Design review of the part built by this model. Coordinates are the model's own, in mm. Face numbers are marked on the shaded views. A direction names the side the tool comes from. Give positions to 0.01 mm unless a question says otherwise; leave off trailing zeros. Write each loop counter-clockwise with the first axis right and the second up, starting at its lowest first coordinate (ties: lowest second). Pieces come first, ordered by that corner, then holes.
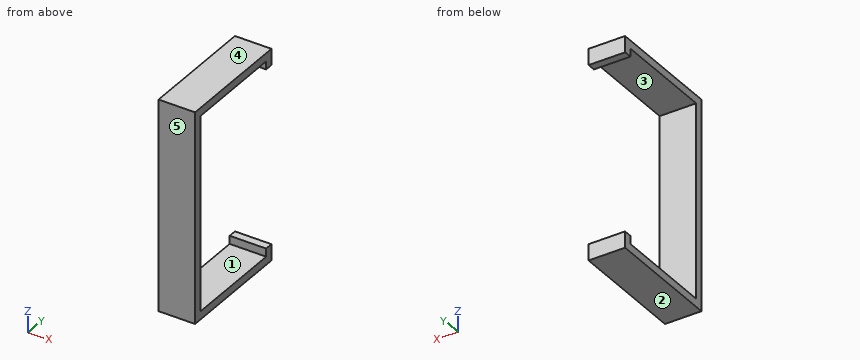
Autodesk Inventor part; units mm, degrees
ref_plane "YZ Plane" through (0, 0, 0) normal (1, 0, 0) x (0, 1, 0)
ref_plane "XZ Plane" through (0, 0, 0) normal (0, 1, 0) x (-1, 0, 0)
ref_plane "XY Plane" through (0, 0, 0) normal (0, 0, 1) x (1, 0, 0)
sketch "Skizze1" plane through (0, 0, 0) normal (0, 1, 0) x (-1, 0, 0)
  line L0 (0, 0) -> (12, 0)
  line L1 (12, 0) -> (12, -26)
  line L2 (12, -26) -> (0, -26)
  line L3 (0, -26) -> (0, 0)
  dimension "d0" = 12
  dimension "d1" = 26
extrude "Extrusion1" add sketch "Skizze1" along normal blind 1
sketch "Skizze2" plane through (0, 0, 0) normal (1, 0, 0) x (0, 0, -1)
  line L0 (26, 1) -> (0, 1)
  line L1 (0, 1) -> (0, 14.5)
  line L2 (0, 1) -> (13.5, 1) construction
  line L3 (0, 14.5) -> (2, 14.5)
  line L4 (2, 14.5) -> (2, 13.5)
  line L5 (2, 13.5) -> (1, 13.5)
  line L6 (1, 13.5) -> (1, 1)
  line L7 (0, 1) -> (1, 1)
  line L8 (24, 14.5) -> (26, 14.5)
  line L9 (26, 14.5) -> (26, 1)
  line L10 (26, 1) -> (25, 1)
  line L11 (25, 1) -> (25, 13.5)
  line L12 (25, 13.5) -> (24, 13.5)
  line L13 (24, 13.5) -> (24, 14.5)
  line L14 (25, 1) -> (26, 1)
  line L15 (26, 0) -> (26, 1)
  point P0 (0, 0)
  dimension "d4" = 13.5
  dimension "d5" = 90
  dimension "d6" = 2
  dimension "d7" = 1
  dimension "d8" = 1
  dimension "d9" = 2
  dimension "d10" = 24
  dimension "d11" = 1
  dimension "d12" = 13.5
  dimension "d13" = 0
extrude "Extrusion2" add sketch "Skizze2" against normal blind 12
sketch "Skizze3" plane through (-12, 0, 0) normal (0, 0, 1) x (1, 0, 0)
  line L0 (0, 0) -> (0, 14.5)
  line L1 (0, 0) -> (4, 0)
  line L2 (4, 0) -> (4, 1)
  line L3 (4, 1) -> (0, 1)
  line L4 (0, 1) -> (0, 0)
  line L5 (12, 14.5) -> (0, 14.5)
  line L6 (5, 14.5) -> (7.5, 14.5)
  line L7 (7.5, 14.5) -> (7.5, 1)
  line L8 (5, 14.5) -> (5, 1)
  line L9 (5, 1) -> (7.5, 1)
  line L10 (12, 0) -> (12, 14.5)
  dimension "d16" = 4
  dimension "d17" = 1
  dimension "d18" = 2.5
  dimension "d19" = 13.5
  dimension "d20" = 13.5
  dimension "d21" = 2.5
  dimension "d22" = 90
  dimension "d23" = 4.5
extrude "Extrusion3" cut sketch "Skizze3" against normal blind 26.5
sketch "Skizze4" plane through (0, 0, 0) normal (0, 0, 1) x (1, 0, 0)
  line L0 (-4.5, 1) -> (-4.5, 14.5)
  line L1 (-4.5, 14.5) -> (-16.7717, 14.5)
  line L2 (-16.7717, 14.5) -> (-16.7717, 0)
  line L3 (-16.7717, 0) -> (-4.5, 0)
  line L4 (-4.5, 0) -> (-4.5, 14.5)
  point P0 (0, 0)
extrude "Extrusion4" cut sketch "Skizze4" against normal blind 26.5
equation "\"Biegeradius\" = Stärke"
equation "\"BreiteBiegungsfreistellung\" = Stärke"
equation "\"TiefeBiegungsfreistellung\" = 0.5 * Stärke"
equation "\"GrößeEckenfreistellung\" = 4 * Stärke"
equation "\"MinimalRest\" = 2 * Stärke"
equation "\"Übergangsradius\" = Biegeradius"
equation "\"JacobiRadiusGröße\" = Biegeradius"
equation "\"Abstandsgröße\" = Stärke"
properties part number "ServoHalterung_unten"
(1) Mouldability with a two-part tool opening along Y and no side actions: class the marked faces 3, 4 and 5 as pulls with the +Y half, pulls with the -Y half, needs draft (parallel to the pull), parting line crosses it, or undercut.
Resolved:
face 3: undercut
face 4: needs draft
face 5: pulls with the -Y half
(2) Tool access review of the marked faces 1 and 2: name each direction out of +Z, -Z, +X, -X, +Y, -Y from which nothing blocks a thin tool from reaching the whole face with its end or side.
Resolved:
face 1: +X, -X
face 2: -Z, +X, -X, +Y, -Y
(3) To check wall thickness, follow L1, parallel to Z at x = -2.55, y = 2; L2, parallel to Z at x = -1.35, y = 14.25; L3, parallel to Y at x = -3.4, z = -24.25. State the ranges of each line that lie inside material, in increasing order.
Resolved:
L1: z = -26 to -25, -1 to 0
L2: z = -26 to -24, -2 to 0
L3: y = 0 to 1, 13.5 to 14.5
(4) Clearance check with flat-ended pins moving along their axes: P1, Ø1.3, axis at x = -2.5, z = -10, coming from the +Y side; P2, Ø1.3, axis at x = -2.5, y = 7.5, coming from the +Z side; P3, Ø1, axis at y = 7.5, z = -23, coming from the +X side. State where each tip first meets the part, or that it passes through.
Resolved:
P1: stops at y = 1
P2: stops at z = 0
P3: passes through
(5) Consider section A-A, the plane y = 8.5. Give the boundary of the cut face in (x, z).
Resolved:
outline: (-4.5, -26) - (0, -26) - (0, -25) - (-4.5, -25) - close; (-4.5, -1) - (0, -1) - (0, 0) - (-4.5, 0) - close
(6) Consider section C-C, the plane z = -5. Give the boundary of the cut face in (x, y).
Resolved:
outline: (-4.5, 0) - (0, 0) - (0, 1) - (-4.5, 1) - close
(7) Consider section B-B, the plane x = -3.45. Give the boundary of the cut face in (y, z).
Resolved:
outline: (0, -26) - (14.5, -26) - (14.5, -24) - (13.5, -24) - (13.5, -25) - (1, -25) - (1, -1) - (13.5, -1) - (13.5, -2) - (14.5, -2) - (14.5, 0) - (0, 0) - close
